Autodesk Inventor part; units mm, degrees
ref_plane "YZ Plane" through (0, 0, 0) normal (1, 0, 0) x (0, 1, 0)
ref_plane "XZ Plane" through (0, 0, 0) normal (0, 1, 0) x (-1, 0, 0)
ref_plane "XY Plane" through (0, 0, 0) normal (0, 0, 1) x (1, 0, 0)
sketch "Sketch1" plane through (0, 0, 0) normal (1, 0, 0) x (0, 1, 0)
  line L0 (2.5, 0) -> (-2.5, 0)
  line L1 (-2.5, 0) -> (-2.5, -5.1)
  line L2 (-2.5, -5.1) -> (2.5, -5.1)
  line L3 (2.5, -5.1) -> (2.5, 0)
  circle A0 centre (0, -5.1) radius 2.5
  line L4 (0, 0) -> (0, -7.6)
  dimension "d0" = 5
  dimension "d1" = 5.1
revolve "Revolution1" add sketch "Sketch1" angle 360 about axis through (0, 0, 0) along (0, 0, -1) picked at (1.6458, -5.2854) picked at (1.6458, -4.9146) contours L3 A0 L4 L0 | A0 L4 L2 | L2 L4 A0
sketch "Sketch2" plane through (0, 0, 0) normal (0, 0, 1) x (1, 0, 0)
  line L0 (-1, -0.5) -> (-2, -0.5)
  line L1 (-2, -0.5) -> (-2, 0.5)
  line L2 (-2, 0.5) -> (-1, 0.5)
  line L3 (-1, 0.5) -> (-1, -0.5)
  line L4 (2, -0.5) -> (1, -0.5)
  line L5 (1, -0.5) -> (1, 0.5)
  line L6 (1, 0.5) -> (2, 0.5)
  line L7 (2, 0.5) -> (2, -0.5)
  point P0 (0, 0)
  point P1 (1, 0)
  dimension "d3" = 1
  dimension "d4" = 1
  dimension "d5" = 1
  dimension "d6" = 2
  dimension "d7" = 1
extrude "Extrusion1" add sketch "Sketch2" along normal blind 25.4
properties part number "LED" material "PC/ABS Plastic"
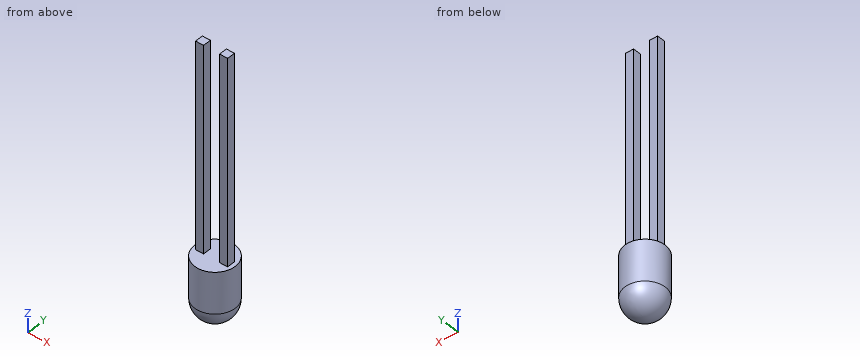
The model under review builds one solid part; all positions refer to its coordinate system, in mm. Round coordinates to 2 decimals unless told otherwise and drop trailing zeros. Loops run counter-clockwise (first coordinate to the right, second up) from the corner with the lowest first, then second, coordinate; pieces in that order, holes last. Notation, with made-up numbers: (-14.75, -38.75) -> (-5.75, -38.75) arc R20 cw to (-5.75, -21.75) -> close; hole circle Ø2 at (82, 67). An arc over 180 degrees is marked (long way). Return JSON: item names as keys, results as strings.
(1) Add section D-D on z = -4. Write out the cut boundary in (x, y).
Solved:
{"outline": "circle Ø5 at (0, 0)"}
(2) Add section A-A on z = 18.5. Write out the cut boundary in (x, y), plus the area to 3 significant figures.
Solved:
{"outline": "(-2, -0.5) -> (-1, -0.5) -> (-1, 0.5) -> (-2, 0.5) -> close; (1, -0.5) -> (2, -0.5) -> (2, 0.5) -> (1, 0.5) -> close", "area": "2.00 mm2"}
(3) For pin 1 (0.5 mm diameter, centred on y = 0, z = 7, fed in from -X); pin 2 (1.5 mm diameter, centred on x = 0, y = -0.5, fed in from +Z); pin 3 (0.8 mm diameter, centred on x = -1.5, z = 18, fed in from +Y), all flat-tipped, find the tip position at first contact; note any pin that passes through.
Solved:
{"pin 1": "x = -2", "pin 2": "z = 0", "pin 3": "y = 0.5"}
(4) Add section C-C on x = -1.4. Write out the cut boundary in (y, z).
Solved:
{"outline": "(-2.07, -5.1) arc R2.07 ccw to (2.07, -5.1) -> (2.07, 0) -> (0.5, 0) -> (0.5, 25.4) -> (-0.5, 25.4) -> (-0.5, 0) -> (-2.07, 0) -> close"}
(5) Add section B-B on y = 0. Write out the cut boundary in (x, z), plus the area to 3 significant figures.
Solved:
{"outline": "(-2.5, -5.1) arc R2.5 ccw to (2.5, -5.1) -> (2.5, 0) -> (2, 0) -> (2, 25.4) -> (1, 25.4) -> (1, 0) -> (-1, 0) -> (-1, 25.4) -> (-2, 25.4) -> (-2, 0) -> (-2.5, 0) -> close", "area": "86.1 mm2"}
(6) For line 1 (X direction, y = 0, z = 12.5); line 2 (Y direction, x = -1.75, z = 23); line 3 (Y direction, x = 0.15, z = -1), list the stretches that pass through material, from the lowest coordinate up.
Solved:
{"line 1": "-2 to -1, 1 to 2", "line 2": "-0.5 to 0.5", "line 3": "-2.5 to 2.5"}
